Geometry check sheet. Reference: the model listing, model coordinates, mm. Face numbers are marked on the shaded views. Coordinates: 2 decimals unless noted, no trailing zeros. Write each loop counter-clockwise with the first axis right and the second up, starting at its lowest first coordinate (ties: lowest second). Pieces come first, ordered by that corner, then holes. Notation, with made-up numbers: (64.5, 21.5) -> (81.5, 21.5) arc R20 ccw to (81.5, 26.5) -> close; hole circle Ø5 at (36, 60.5). An arc over 180 degrees is marked (long way). Answer as CSV lines item,"result".
```python
from build123d import *

# Parameters (mm, degrees)
BOSS_EXTRUDE1_DEPTH     = 0.5
BOSS_EXTRUDE2_DEPTH     = 4
FILLET1_R               = 0.2
CUT_EXTRUDE1_DEPTH      = 32.104662098
CUT_EXTRUDE1_DEPTH_BACK = 32.104662098
SKETCH3_R               = 3.03


with BuildPart() as part:
    # Sketch1 → Boss-Extrude1 (new body)
    with BuildSketch(Plane(origin=(0, 0, 0), x_dir=(1, 0, 0), z_dir=(0, 1, 0))):
        with BuildLine():
            Line((-19, 17.5), (-19, -17.5))
            ThreePointArc((-19, -17.5), (-18.267766953, -19.267766953), (-16.5, -20))
            Line((-16.5, -20), (16.5, -20))
            ThreePointArc((16.5, -20), (18.267766953, -19.267766953), (19, -17.5))
            Line((19, -17.5), (19, 17.5))
            ThreePointArc((19, 17.5), (18.267766953, 19.267766953), (16.5, 20))
            Line((16.5, 20), (-16.5, 20))
            ThreePointArc((-16.5, 20), (-18.267766953, 19.267766953), (-19, 17.5))
        make_face()
    extrude(amount=BOSS_EXTRUDE1_DEPTH)

    # Sketch2 → Boss-Extrude2 (add)
    with BuildSketch(Plane(origin=(0, 0.5, 0), x_dir=(1, 0, 0), z_dir=(0, 1, 0))):
        with BuildLine():
            Line((-19.5, 22.5), (19.5, 22.5))
            ThreePointArc((19.5, 22.5), (20.560660172, 22.060660172), (21, 21))
            Line((21, 21), (21, 19.314104738))
            ThreePointArc((21, 19.314104738), (20.532, 17.5), (21, 15.685895262))
            Line((21, 15.685895262), (21, -15.685895262))
            ThreePointArc((21, -15.685895262), (20.532, -17.5), (21, -19.314104738))
            Line((21, -19.314104738), (21, -21))
            ThreePointArc((21, -21), (20.560660172, -22.060660172), (19.5, -22.5))
            Line((19.5, -22.5), (-19.5, -22.5))
            ThreePointArc((-19.5, -22.5), (-20.560660172, -22.060660172), (-21, -21))
            Line((-21, -21), (-21, -19.314104738))
            ThreePointArc((-21, -19.314104738), (-20.532, -17.5), (-21, -15.685895262))
            Line((-21, -15.685895262), (-21, 15.685895262))
            ThreePointArc((-21, 15.685895262), (-20.532, 17.5), (-21, 19.314104738))
            Line((-21, 19.314104738), (-21, 21))
            ThreePointArc((-21, 21), (-20.560660172, 22.060660172), (-19.5, 22.5))
        make_face()
    extrude(amount=BOSS_EXTRUDE2_DEPTH)

    # Fillet1
    fillet1_edges = [part.edges().sort_by_distance(p)[0] for p in [
        (0, 0, 20),
        (-18.267766953, 0, 19.267766953),
        (-20.532, 0.5, 17.5),
        (-21, 0.5, 20.157052369),
        (-20.560660172, 0.5, 22.060660172),
        (0, 0.5, 22.5),
        (20.560660172, 0.5, 22.060660172),
        (21, 0.5, 20.157052369),
        (20.532, 0.5, 17.5),
        (21, 0.5, 0),
        (20.532, 0.5, -17.5),
        (21, 0.5, -20.157052369),
        (20.560660172, 0.5, -22.060660172),
        (0, 0.5, -22.5),
        (-20.560660172, 0.5, -22.060660172),
        (-21, 0.5, -20.157052369),
        (-20.532, 0.5, -17.5),
        (-21, 0.5, 0),
        (-19, 0, 0),
        (-18.267766953, 0, -19.267766953),
        (0, 0, -20),
        (18.267766953, 0, -19.267766953),
        (19, 0, 0),
        (18.267766953, 0, 19.267766953),
    ]]
    fillet(fillet1_edges, radius=FILLET1_R)

    # Sketch3 → Cut-Extrude1 (cut, two sides: drawn at the far end of the back side and taken through both)
    with BuildSketch(Plane.XY.offset(-CUT_EXTRUDE1_DEPTH_BACK)):
        with Locations((9.75, 4.78)):
            Circle(SKETCH3_R)
        with Locations((3.25, 4.78)):
            Circle(SKETCH3_R)
        with Locations((-3.25, 4.78)):
            Circle(SKETCH3_R)
        with Locations((-9.75, 4.78)):
            Circle(SKETCH3_R)
    extrude(amount=CUT_EXTRUDE1_DEPTH + CUT_EXTRUDE1_DEPTH_BACK, mode=Mode.SUBTRACT)


solid = part.part
```
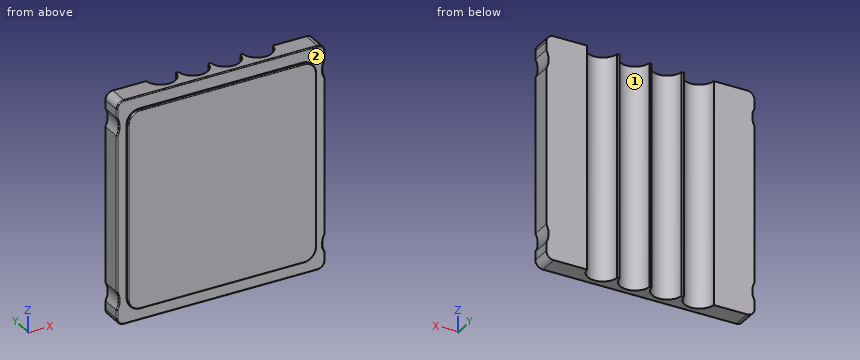
Item 1: Depth check by flat-ended pin: pin 1 Ø2 at (y, z) = (2, -16) entering from +X. Enter the tip coordinate at first touch or a pass-through.
Responses:
pin 1,"stops at x = 21"
Item 2: Thickness scan on probe 1 along X at (y, z) = (2.4, 6.5); probe 2 along X at (y, z) = (3.55, -14); probe 3 along Z at (x, y) = (3, 0.3). Record the ranges inside material, lowest first.
Responses:
probe 1,"x = -21 to -11.63, -7.87 to -5.13, -1.37 to 1.37, 5.13 to 7.87, 11.63 to 21"
probe 2,"x = -21 to -12.52, -6.98 to -6.02, -0.48 to 0.48, 6.02 to 6.98, 12.52 to 21"
probe 3,"z = -20 to 20"
Item 3: Cross-section at C-C, the plane x = -11. Record the cut outline in (y, z).
Responses:
outline,"(0, -19.8) arc R0.2 ccw to (0.2, -20) -> (0.5, -20) -> (0.5, -22.3) arc R0.2 ccw to (0.7, -22.5) -> (2.02, -22.5) -> (2.02, 22.5) -> (0.7, 22.5) arc R0.2 ccw to (0.5, 22.3) -> (0.5, 20) -> (0.2, 20) arc R0.2 ccw to (0, 19.8) -> close"
Item 4: Cross-section at B-B, the plane z = -14. Record the cut outline in (x, y), plus the area to 3 significant figures.
Responses:
outline,"(-21, 0.7) arc R0.2 ccw to (-20.8, 0.5) -> (-19, 0.5) -> (-19, 0.2) arc R0.2 ccw to (-18.8, 0) -> (18.8, 0) arc R0.2 ccw to (19, 0.2) -> (19, 0.5) -> (20.8, 0.5) arc R0.2 ccw to (21, 0.7) -> (21, 4.5) -> (12.77, 4.5) arc R3.03 cw to (6.73, 4.5) -> (6.27, 4.5) arc R3.03 cw to (0.23, 4.5) -> (-0.23, 4.5) arc R3.03 cw to (-6.27, 4.5) -> (-6.73, 4.5) arc R3.03 cw to (-12.77, 4.5) -> (-21, 4.5) -> close"
area,"136 mm2"
Item 5: Cross-section at D-D, the plane x = 1. Record the cut outline in (y, z), plus the area to 3 significant figures.
Responses:
outline,"(0, -19.8) arc R0.2 ccw to (0.2, -20) -> (0.5, -20) -> (0.5, -22.3) arc R0.2 ccw to (0.7, -22.5) -> (2.75, -22.5) -> (2.75, 22.5) -> (0.7, 22.5) arc R0.2 ccw to (0.5, 22.3) -> (0.5, 20) -> (0.2, 20) arc R0.2 ccw to (0, 19.8) -> close"
area,"121 mm2"
Item 6: Cross-section at A-A, the plane y = 3.25. Count the separate pieces of the cut face and the enclosed holes in it, plus the area to 3 significant figures.
Responses:
separate pieces,"5"
enclosed holes,"0"
area,"942 mm2"
Item 7: Release check for a two-part mould opening along X. For the marked faces 1 and 2 record: +X half, -X half, draft (parallel to the pull), parting line (faces both ways), or undercut.
Responses:
face 1,"undercut"
face 2,"draft"
